from build123d import *

# Parameters (mm, degrees)
SKETCH1_R            = 3.95
BOSS_EXTRUDE1_DEPTH  = 28
BOSS_EXTRUDE2_START  = 8
BOSS_EXTRUDE2_DEPTH  = 8
SKETCH3_R            = 5
BOSS_EXTRUDE3_DEPTH  = 3
SKETCH5_W            = 3.2
SKETCH5_H            = 7.25
CUT_EXTRUDE1_DEPTH   = 42
M4_CLEARANCE_HOLE1_D = 4.5
CHAMFER1_SIZE        = 0.5
FILLET1_R            = 3.7
FILLET5_R            = 6


with BuildPart() as part:
    # Sketch1 → Boss-Extrude1 (new body)
    with BuildSketch(Plane.XY):
        Circle(SKETCH1_R)
    extrude(amount=-BOSS_EXTRUDE1_DEPTH)

    # Sketch2 → Boss-Extrude2 (add)
    with BuildSketch(Plane.XY.offset(BOSS_EXTRUDE2_START)):
        with BuildLine():
            ThreePointArc((6.35, 0), (5.708717799, 2.780834604), (3.914396505, 5))
            Line((3.914396505, 5), (0, 5))
            Line((0, 5), (0, 3.95))
            ThreePointArc((0, 3.95), (2.793071786, 2.793071786), (3.95, 0))
            ThreePointArc((3.95, 0), (2.793071786, -2.793071786), (0, -3.95))
            Line((0, -3.95), (0, -5))
            Line((0, -5), (3.914396505, -5))
            ThreePointArc((3.914396505, -5), (5.708717799, -2.780834604), (6.35, 0))
        make_face()
        with BuildLine():
            Line((0, 5), (3.914396505, 5))
            ThreePointArc((3.914396505, 5), (-6.35, 0), (3.914396505, -5))
            Line((3.914396505, -5), (0, -5))
            Line((0, -5), (0, -3.95))
            ThreePointArc((0, -3.95), (-3.95, 0), (0, 3.95))
            Line((0, 3.95), (0, 5))
        make_face()
        with BuildLine():
            Line((145, -5), (145, 5))
            Line((145, 5), (3.914396505, 5))
            ThreePointArc((3.914396505, 5), (5.708717799, 2.780834604), (6.35, 0))
            ThreePointArc((6.35, 0), (5.708717799, -2.780834604), (3.914396505, -5))
            Line((3.914396505, -5), (145, -5))
        make_face()
        with BuildLine():
            ThreePointArc((3.95, 0), (2.793071786, 2.793071786), (0, 3.95))
            Line((0, 3.95), (0, -3.95))
            ThreePointArc((0, -3.95), (2.793071786, -2.793071786), (3.95, 0))
        make_face()
        with BuildLine():
            Line((0, -3.95), (0, 3.95))
            ThreePointArc((0, 3.95), (-3.95, 0), (0, -3.95))
        make_face()
    extrude(amount=-BOSS_EXTRUDE2_DEPTH)

    # Sketch3 → Boss-Extrude3 (add)
    with BuildSketch(Plane.XY):
        Circle(SKETCH3_R)
    extrude(amount=-BOSS_EXTRUDE3_DEPTH)

    # Sketch5 → Cut-Extrude1 (cut)
    with BuildSketch(Plane(origin=(145, 0, 0), x_dir=(0, 0, -1), z_dir=(1, 0, 0))):
        with Locations((-1.6, 0)):
            Rectangle(SKETCH5_W, SKETCH5_H)
    extrude(amount=-CUT_EXTRUDE1_DEPTH, mode=Mode.SUBTRACT)

    # M4 Clearance Hole1 (through all)
    with Locations(Plane.XY.offset(8)):
        with Locations((140, 0), (130, 0), (120, 0), (110, 0)):
            Hole(M4_CLEARANCE_HOLE1_D / 2)

    # Chamfer1
    chamfer1_edges = [part.edges().sort_by_distance(p)[0] for p in [
        (-3.95, 0, -28),
    ]]
    chamfer(chamfer1_edges, length=CHAMFER1_SIZE)

    # Fillet1
    # the kernel refuses this fillet: 3.7 mm, written as the material it adds along each edge
    with BuildSketch(Plane(origin=(103, -3.625, 3.2), x_dir=(0, 1, 0), z_dir=(0, 0, -1))) as fillet1_piece_1:
        with BuildLine():
            CenterArc((FILLET1_R, FILLET1_R), FILLET1_R, 180, 90)
            Line((0, FILLET1_R), (0, 0))
            Line((0, 0), (FILLET1_R, 0))
        make_face()
    extrude(amount=3.2)
    with BuildSketch(Plane(origin=(103, 3.625, 0), x_dir=(1, 0, 0), z_dir=(0, 0, 1))) as fillet1_piece_2:
        with BuildLine():
            CenterArc((FILLET1_R, -FILLET1_R), FILLET1_R, 90, 90)
            Line((0, -FILLET1_R), (0, 0))
            Line((0, 0), (FILLET1_R, 0))
        make_face()
    extrude(amount=3.2)

    # Fillet5
    fillet5_edges = [part.edges().sort_by_distance(p)[0] for p in [
        (145, 4.3125, 0),
    ]]
    fillet(fillet5_edges, radius=FILLET5_R)


solid = part.part
Verification items for the finished model (mm, model axes). A direction names the side the tool comes from. Round coordinates to 2 decimals unless told otherwise and drop trailing zeros. Loops run counter-clockwise (first coordinate to the right, second up) from the corner with the lowest first, then second, coordinate; pieces in that order, holes last. Notation, with made-up numbers: M 87.25,40 L 110.25,40 A19 cw 110.25,57 Z; hole C 54,53 d10. An arc over 180 degrees is marked long. Write each question's results on one line, items separated by ' | '.
1) Scan lines: L1, parallel to Y at x = 140, z = 4.35; L2, parallel to Z at x = 78, y = 1; L3, parallel to Y at x = 49.5, z = 1. Record each from-to range of solid material in increasing order. Write a range as from..to.
Checks:
L1: y = -5..-2.25, 2.25..5 | L2: z = 0..8 | L3: y = -5..5
2) Section check C-C on z = -19. Record the boundary of the cut face in (x, y).
Checks:
outline: C 0,0 d7.9
3) Section check D-D on x = 80. Record the boundary of the cut face in (y, z), then the cut area to 3 significant figures.
Checks:
outline: M -5,0 L 5,0 L 5,8 L -5,8 Z | area: 80.0 mm2
4) Mould release check, pull along Y, two halves, no side actions. Record for faces 1 (the cylindrical face through (104.139, 2.596, 1.578)), 2 (the flat face through (0, 0, -28)), 3 (the cylindrical face through (-6.347, 0.199, 4.056)): released by +Y, released by -Y, zero draft, split by the parting line, or undercut.
Checks:
face 1: undercut | face 2: zero draft | face 3: split by the parting line
5) Gauge pin test, flat ends, axial feed: P1, Ø12, axis at x = 42, z = -10, coming from the -Y side; P2, Ø6, axis at x = 43, z = 1.5, coming from the +Y side; P3, Ø6, axis at x = 120, y = 0, coming from the -Z side; P4, Ø12, axis at x = 78, z = -1, coming from the -Y side. Record the tip position at first contact, or that the pin passes through.
Checks:
P1: passes through | P2: stops at y = 5 | P3: stops at z = 3.2 | P4: stops at y = -5
6) Section check A-A on x = 130. Record the boundary of the cut face in (y, z) (3 decimals).
Checks:
outline: M -5,0 L -3.625,0 L -3.625,3.2 L -2.25,3.2 L -2.25,8 L -5,8 Z; M 2.25,3.2 L 3.625,3.2 L 3.625,0 L 5,0 L 5,8 L 2.25,8 Z
7) Section check B-B on x = 0. Record the boundary of the cut face in (y, z).
Checks:
outline: M -6.35,0 L -5,0 L -5,-3 L -3.95,-3 L -3.95,-27.5 L -3.45,-28 L 3.45,-28 L 3.95,-27.5 L 3.95,-3 L 5,-3 L 5,0 L 6.35,0 L 6.35,8 L -6.35,8 Z
8) Access from +Z, -Z, +X, -X, +Y, -Y to the whole of each face (thin tool, end or side, straight path). Record for faces 4 (the cylindrical face through (-1.08, -4.88, -1.48)), 5 (the flat face through (75, 5, 4)), 6 (the flat face through (126, -3.625, 2)).
Checks:
face 4: -Z | face 5: +Z, -Z, +X, +Y | face 6: -Z, +X
